```python
from build123d import *

# Parameters (mm, degrees)
SKETCH2_W       = 47.752
SKETCH2_H       = 4.7625
LPATTERN1_COUNT = 4
LPATTERN1_PITCH = 3.6068
SKETCH6_W       = 4.7625
SKETCH6_H       = 27.2415
LPATTERN2_COUNT = 4
LPATTERN2_PITCH = 3.6068
SKETCH9_W       = 1.6256
SKETCH9_H       = 27.2415
CHAMFER1_SIZE   = 0.127
FILLET1_R       = 0.127


with BuildPart() as part:
    # Sketch2 → Revolve1 (revolve)
    with BuildSketch(Plane(origin=(0, 0, 0), x_dir=(0, 0, -1), z_dir=(1, 0, 0)), mode=Mode.PRIVATE) as revolve1_sk:
        with Locations((0, 2.38125)):
            Rectangle(SKETCH2_W, SKETCH2_H)
    revolve(revolve1_sk.sketch.rotate(Axis((0, 0, 23.876), (0, 0, -1)), 90), axis=Axis((0, 0, 23.876), (0, 0, -1)))

    # Sketch3 → Cut-Revolve1 (revolve, cut)
    with BuildSketch(Plane(origin=(0, 0, 0), x_dir=(0, 0, -1), z_dir=(1, 0, 0)), mode=Mode.PRIVATE) as cut_revolve1_sk:
        Polygon((-23.876, 4.7625), (-23.876, 2.38125), (-9.4488, 2.38125), (-5.842, 2.921), (-5.842, 4.7625), align=None)
    cut_revolve1 = revolve(cut_revolve1_sk.sketch.rotate(Axis((0, 0, 23.876), (0, 0, -1)), 90), axis=Axis((0, 0, 23.876), (0, 0, -1)), mode=Mode.SUBTRACT)

    # Sketch4 → Revolve2 (revolve)
    with BuildSketch(Plane(origin=(0, 0, 0), x_dir=(0, 0, -1), z_dir=(1, 0, 0))):
        Polygon((-20.2692, 2.921), (-20.3962, 2.921), (-23.876, 2.38125), (-20.2692, 2.38125), align=None)
    revolve2 = revolve(axis=Axis((0, 0, 5.842), (0, 0, 1)))

    # LPattern1: Revolve2 ×4
    with Locations(*[(0, 0, -i * LPATTERN1_PITCH) for i in range(1, LPATTERN1_COUNT)]):
        add(revolve2)

    # Mirror1: Cut-Revolve1, Revolve2 across plane
    add(cut_revolve1.mirror(Plane.XY), mode=Mode.SUBTRACT)
    add(revolve2.mirror(Plane.XY))

    # Mirror1 copy 1 sketch → Mirror1 copy 1 (revolve)
    with BuildSketch(Plane(origin=(0, 0, 3.6068), x_dir=(0, 0, 1), z_dir=(1, 0, 0))):
        Polygon((-20.2692, -2.921), (-20.3962, -2.921), (-23.876, -2.38125), (-20.2692, -2.38125), align=None)
    revolve(axis=Axis((0, 0, -2.2352), (0, 0, 1)))

    # Mirror1 copy 2 sketch → Mirror1 copy 2 (revolve)
    with BuildSketch(Plane(origin=(0, 0, 7.2136), x_dir=(0, 0, 1), z_dir=(1, 0, 0))):
        Polygon((-20.2692, -2.921), (-20.3962, -2.921), (-23.876, -2.38125), (-20.2692, -2.38125), align=None)
    revolve(axis=Axis((0, 0, 1.3716), (0, 0, 1)))

    # Mirror1 copy 3 sketch → Mirror1 copy 3 (revolve)
    with BuildSketch(Plane(origin=(0, 0, 10.8204), x_dir=(0, 0, 1), z_dir=(1, 0, 0))):
        Polygon((-20.2692, -2.921), (-20.3962, -2.921), (-23.876, -2.38125), (-20.2692, -2.38125), align=None)
    revolve(axis=Axis((0, 0, 4.9784), (0, 0, 1)))

    # Sketch6 → Revolve3 (revolve)
    with BuildSketch(Plane(origin=(0, 0, 0), x_dir=(0, 0, -1), z_dir=(1, 0, 0)), mode=Mode.PRIVATE) as revolve3_sk:
        with Locations((-2.38125, 13.62075)):
            Rectangle(SKETCH6_W, SKETCH6_H)
    revolve(revolve3_sk.sketch.rotate(Axis((0, 0, 0), (0, 1, 0)), 180), axis=Axis((0, 0, 0), (0, 1, 0)))

    # Sketch7 → Cut-Revolve3 (revolve, cut)
    with BuildSketch(Plane(origin=(0, 0, 0), x_dir=(0, 0, -1), z_dir=(1, 0, 0)), mode=Mode.PRIVATE) as cut_revolve3_sk:
        Polygon((-2.921, 9.2075), (-2.38125, 12.8143), (-2.38125, 27.2415), (-4.7625, 27.2415), (-4.7625, 9.2075), align=None)
    revolve(cut_revolve3_sk.sketch.rotate(Axis((0, 0, 0), (0, 1, 0)), 180), axis=Axis((0, 0, 0), (0, 1, 0)), mode=Mode.SUBTRACT)

    # Sketch8 → Revolve4 (revolve)
    with BuildSketch(Plane(origin=(0, 0, 0), x_dir=(0, 0, -1), z_dir=(1, 0, 0)), mode=Mode.PRIVATE) as revolve4_sk:
        Polygon((-2.38125, 27.2415), (-2.921, 23.7617), (-2.921, 23.6347), (-2.38125, 23.6347), align=None)
    revolve4 = revolve(revolve4_sk.sketch.rotate(Axis((0, 27.2415, 0), (0, -1, 0)), 180), axis=Axis((0, 27.2415, 0), (0, -1, 0)))

    # LPattern2: Revolve4 ×4
    with Locations(*[(0, -i * LPATTERN2_PITCH, 0) for i in range(1, LPATTERN2_COUNT)]):
        add(revolve4)

    # Sketch5 → Cut-Revolve2 (revolve, cut)
    with BuildSketch(Plane(origin=(0, 0, 0), x_dir=(0, 0, -1), z_dir=(1, 0, 0))):
        with BuildLine():
            Line((-23.876, 1.6256), (0, 1.6256))
            ThreePointArc((0, 1.6256), (1.149472783, 1.149472783), (1.6256, 0))
            Line((1.6256, 0), (-23.876, 0))
            Line((-23.876, 0), (-23.876, 1.6256))
        make_face()
    revolve(axis=Axis((0, 0, 23.876), (0, 0, -1)), mode=Mode.SUBTRACT)

    # Sketch9 → Cut-Revolve4 (revolve, cut)
    with BuildSketch(Plane(origin=(0, 0, 0), x_dir=(0, 0, -1), z_dir=(1, 0, 0))):
        with Locations((-0.8128, 13.62075)):
            Rectangle(SKETCH9_W, SKETCH9_H)
    revolve(axis=Axis((0, 27.2415, 0), (0, -1, 0)), mode=Mode.SUBTRACT)

    # Chamfer1
    chamfer1_edges = [part.edges().sort_by_distance(p)[0] for p in [
        (-4.7625, 0, -5.842),
        (0, 9.2075, 4.7625),
        (-4.7625, 0, 5.842),
    ]]
    chamfer(chamfer1_edges, length=CHAMFER1_SIZE)

    # Fillet1
    fillet1_edges = [part.edges().sort_by_distance(p)[0] for p in [
        (0, -2.38125, 23.876),
        (0, -2.38125, -23.876),
        (0, 27.2415, 2.38125),
    ]]
    fillet(fillet1_edges, radius=FILLET1_R)


solid = part.part
```
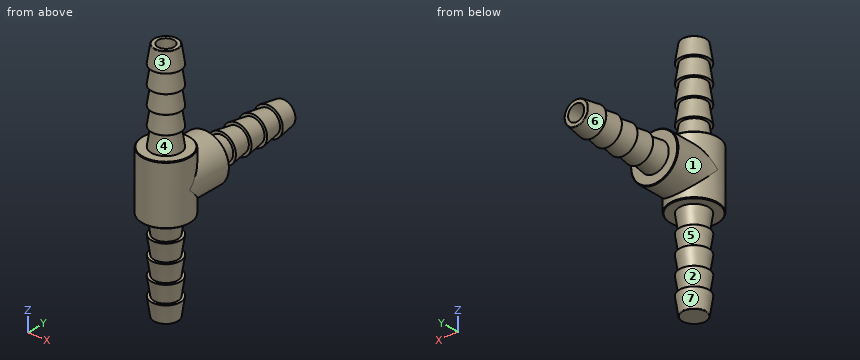
Geometry check sheet. Reference: the model listing, model coordinates, mm. Face numbers are marked on the shaded views. A direction names the side the tool comes from. Round coordinates to 2 decimals unless told otherwise and drop trailing zeros. Order: outer loops, then holes, each group sorted by start corner. A loop starts at its lowest first (then second) coordinate and runs counter-clockwise, first axis right, second up. Notation, with made-up numbers: M -36,82 L 19,82 A28 ccw 19,110 Z; hole C 75.5,51 d10. An arc over 180 degrees is marked long. Answer as CSV lines item,"result".
1) Sectioned sample at A-A on y = 5.5. Record the cut outline in (x, z) (1 decimal), and give its area (3 significant figures).
Entries:
outline,"C 0,0 d9.5; hole C 0,0 d3.3"
area,"63.0 mm2"
2) Gauge pin test, flat ends, axial feed: pin 1 Ø1.5 at (x, z) = (-2, -3) entering from -Y; pin 2 Ø10 at (y, z) = (14.5, -12) entering from -X; pin 3 Ø1 at (x, y) = (-1, 19) entering from -Z; pin 4 Ø1.5 at (y, z) = (3, 8) entering from -X. Record the tip position at first contact, or that the pin passes through.
Entries:
pin 1,"y = -4.6"
pin 2,"through"
pin 3,"z = -2.52"
pin 4,"x = -1.32"
3) Sectioned sample at B-B on z = 10.5. Record the cut outline in (x, y), and give its area (3 significant figures).
Entries:
outline,"C 0,0 d5.56; hole C 0,0 d3.25"
area,"15.9 mm2"
4) Tool access check on the marked faces 1, 2 and 3. Record the directions out of +Z, -Z, +X, -X, +Y, -Y that give a thin tool (end or side, any length) a straight path to the whole face; none if there is none.
Entries:
face 1,"+Y"
face 2,"none"
face 3,"+Z"
5) Thickness scan on probe 1 along X at (y, z) = (13, 0); probe 2 along Z at (x, y) = (-2.5, -2); probe 3 along Z at (x, y) = (0, 16.25). Record the ranges inside material, lowest first. Write a range as [from, to].
Entries:
probe 1,"[-2.91, -1.63], [1.63, 2.91]"
probe 2,"[-5.84, 5.84]"
probe 3,"[-2.41, -1.63], [1.63, 2.41]"
6) Mould release check, pull along Z, two halves, no side actions. Record for the marked faces 4, 5, 6 and 7: +Z half, -Z half, draft (parallel to the pull), parting line (faces both ways), or undercut.
Entries:
face 4,"undercut"
face 5,"undercut"
face 6,"parting line"
face 7,"-Z half"
